from build123d import *

# Parameters (mm, degrees)
IZIM1_W                     = 80
IZIM1_H                     = 20
Y_KSEKLIK_EKSTR_ZYON1_DEPTH = 42
BO_ALTMA1_T                 = -2
IZIM2_R                     = 7.25
KES_EKSTR_ZYON1_DEPTH       = 42


with BuildPart() as part:
    # Çizim1 → Yükseklik-Ekstrüzyon1 (new body)
    with BuildSketch(Plane.XY):
        Rectangle(IZIM1_W, IZIM1_H)
    extrude(amount=Y_KSEKLIK_EKSTR_ZYON1_DEPTH)

    # İç Boşaltma1
    bo_altma1_openings = [part.faces().sort_by_distance(p)[0] for p in [
        (0, 0, 42),
        (0, -10, 21),
        (-40, 0, 21),
        (40, 0, 21),
    ]]
    offset(amount=BO_ALTMA1_T, openings=bo_altma1_openings, kind=Kind.INTERSECTION)

    # Çizim2 → Kes-Ekstrüzyon1 (cut)
    with BuildSketch(Plane(origin=(0, 10, 0), x_dir=(1, 0, 0), z_dir=(0, 1, 0))):
        with Locations((0, -23)):
            Circle(IZIM2_R)
        with Locations((-25, -23)):
            Circle(IZIM2_R)
        with Locations((25, -23)):
            Circle(IZIM2_R)
    extrude(amount=-KES_EKSTR_ZYON1_DEPTH, mode=Mode.SUBTRACT)


solid = part.part
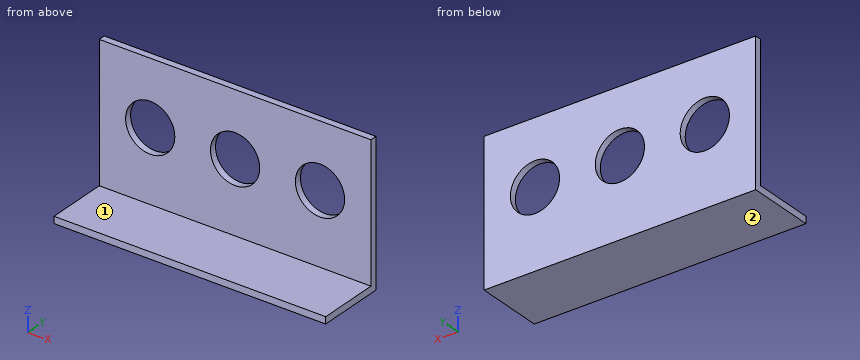
Geometry: final body of the model. Coordinates: model frame, mm. Face numbers are marked on the shaded views. A direction names the side the tool comes from. Give positions to 0.01 mm unless a question says otherwise; leave off trailing zeros. Order: outer loops, then holes, each group sorted by start corner. A loop starts at its lowest first (then second) coordinate and runs counter-clockwise, first axis right, second up. Notation, with made-up numbers: (-18.5, 87) -> (23.5, 87) arc R18 cw to (23.5, 114) -> close; hole circle Ø5 at (31.25, -15.5). An arc over 180 degrees is marked (long way). Put each result on its own line as item: value.
Q1. Pin query (flat end, axial travel): pin 1 (12 mm diameter, centred on x = -7.5, z = 14.5, fed in from -Y); pin 2 (2 mm diameter, centred on y = -5, z = 4.5, fed in from +X); pin 3 (6 mm diameter, centred on x = 17, y = -4.5, fed in from +Z). Return the tip coordinate at first contact, or that it passes through.
Here are the results:
pin 1: stops at y = 8
pin 2: passes through
pin 3: stops at z = 2
Q2. Section A-A, the plane z = 23. Return loops of the section in (x, y), then the cut area to 3 significant figures.
Here are the results:
outline: (-40, 8) -> (-32.25, 8) -> (-32.25, 10) -> (-40, 10) -> close; (-17.75, 8) -> (-7.25, 8) -> (-7.25, 10) -> (-17.75, 10) -> close; (7.25, 8) -> (17.75, 8) -> (17.75, 10) -> (7.25, 10) -> close; (32.25, 8) -> (40, 8) -> (40, 10) -> (32.25, 10) -> close
area: 73.0 mm^2
Q3. Section C-C, the plane y = 8.75. Return loops of the section in (x, z), then the cut area to 3 significant figures.
Here are the results:
outline: (-40, 0) -> (40, 0) -> (40, 42) -> (-40, 42) -> close; hole circle Ø14.5 at (-25, 23); hole circle Ø14.5 at (0, 23); hole circle Ø14.5 at (25, 23)
area: 2,860 mm^2
Q4. Reachability of the marked faces 1 and 2 from +Z, -Z, +X, -X, +Y, -Y: full face, straight path, thin tool, end or side. Return the list, or none.
Here are the results:
face 1: +Z, +X, -X, -Y
face 2: -Z, +X, -X, +Y, -Y
Q5. Section D-D, the plane x = 33. Return loops of the section in (y, z).
Here are the results:
outline: (-10, 0) -> (10, 0) -> (10, 42) -> (8, 42) -> (8, 2) -> (-10, 2) -> close
Q6. Section B-B, the plane x = -25. Return loops of the section in (y, z).
Here are the results:
outline: (-10, 0) -> (10, 0) -> (10, 15.75) -> (8, 15.75) -> (8, 2) -> (-10, 2) -> close; (8, 30.25) -> (10, 30.25) -> (10, 42) -> (8, 42) -> close
Q7. Material intervals for L1, parallel to X at y = 8.85, z = 23; L2, parallel to Z at x = 0, y = 8.8; L3, parallel to Z at x = -20.5, y = -0.25, sorted ascending.
Here are the results:
L1: x = -40 to -32.25, -17.75 to -7.25, 7.25 to 17.75, 32.25 to 40
L2: z = 0 to 15.75, 30.25 to 42
L3: z = 0 to 2
